```python
from build123d import *

# Parameters (mm, degrees)
SKETCH1_W           = 154
SKETCH1_H           = 100
BOSS_EXTRUDE1_DEPTH = 2
SKETCH2_W           = 100
SKETCH2_H           = 2
BOSS_EXTRUDE2_DEPTH = 70
SKETCH3_W           = 90.6
SKETCH3_H           = 8
BOSS_EXTRUDE3_DEPTH = 8
SKETCH4_W           = 10
SKETCH4_H           = 134
BOSS_EXTRUDE4_DEPTH = 8
SKETCH5_W           = 10
SKETCH5_H           = 5
BOSS_EXTRUDE5_DEPTH = 62
SKETCH6_R           = 1.95
CUT_EXTRUDE1_DEPTH  = 195.889943301
SKETCH7_R           = 1.95
CUT_EXTRUDE2_DEPTH  = 195.889943301
FILLET1_R           = 3
SKETCH8_R           = 1.95
CUT_EXTRUDE3_DEPTH  = 15
SKETCH9_R           = 1.95
CUT_EXTRUDE4_DEPTH  = 15
FILLET2_R           = 3


with BuildPart() as part:
    # Sketch1 → Boss-Extrude1 (new body)
    with BuildSketch(Plane(origin=(0, 0, 0), x_dir=(0, 1, 0), z_dir=(0, 0, 1))):
        with Locations((77, 50)):
            Rectangle(SKETCH1_W, SKETCH1_H)
    extrude(amount=BOSS_EXTRUDE1_DEPTH)

    # Sketch2 → Boss-Extrude2 (add)
    with BuildSketch(Plane.XY.offset(2)):
        with Locations((-50, 153)):
            Rectangle(SKETCH2_W, SKETCH2_H)
        with Locations((-50, 1)):
            Rectangle(SKETCH2_W, SKETCH2_H)
    extrude(amount=BOSS_EXTRUDE2_DEPTH)

    # Sketch3 → Boss-Extrude3 (add)
    with BuildSketch(Plane.XY.offset(2)):
        with Locations((-50, 148)):
            Rectangle(SKETCH3_W, SKETCH3_H)
        with Locations((-50, 6)):
            Rectangle(SKETCH3_W, SKETCH3_H)
    extrude(amount=BOSS_EXTRUDE3_DEPTH)

    # Sketch4 → Boss-Extrude4 (add)
    with BuildSketch(Plane.XY.offset(2)):
        with Locations((-50, 77)):
            Rectangle(SKETCH4_W, SKETCH4_H)
    extrude(amount=BOSS_EXTRUDE4_DEPTH)

    # Sketch5 → Boss-Extrude5 (add)
    with BuildSketch(Plane.XY.offset(10)):
        with Locations((-50, 149.5)):
            Rectangle(SKETCH5_W, SKETCH5_H)
        with Locations((-50, 4.5)):
            Rectangle(SKETCH5_W, SKETCH5_H)
    extrude(amount=BOSS_EXTRUDE5_DEPTH)

    # Sketch6 → Cut-Extrude1 (cut, through all)
    with BuildSketch(Plane(origin=(-95.3, 0, 0), x_dir=(0, -1, 0), z_dir=(-1, 0, 0))):
        with Locations((-6, 6)):
            Circle(SKETCH6_R)
    extrude(amount=-CUT_EXTRUDE1_DEPTH, mode=Mode.SUBTRACT)

    # Sketch7 → Cut-Extrude2 (cut, through all)
    with BuildSketch(Plane(origin=(-95.3, 0, 0), x_dir=(0, -1, 0), z_dir=(-1, 0, 0))):
        with Locations(Location((-148, 6, 0), (0, 0, 90))):
            Circle(SKETCH7_R)
    extrude(amount=-CUT_EXTRUDE2_DEPTH, mode=Mode.SUBTRACT)

    # Fillet1
    fillet1_edges = [part.edges().sort_by_distance(p)[0] for p in [
        (-75.15, 144, 10),
        (-24.85, 10, 10),
        (-75.15, 10, 10),
        (-24.85, 144, 10),
        (-55, 77, 10),
        (-45, 77, 10),
    ]]
    fillet(fillet1_edges, radius=FILLET1_R - 0.0001)  # a hair under: the kernel refuses the full size

    # Sketch8 → Cut-Extrude3 (cut)
    with BuildSketch(Plane.XY.offset(72)):
        with Locations((-50, 150)):
            Circle(SKETCH8_R)
    extrude(amount=-CUT_EXTRUDE3_DEPTH, mode=Mode.SUBTRACT)

    # Sketch9 → Cut-Extrude4 (cut)
    with BuildSketch(Plane.XY.offset(72)):
        with Locations((-50, 4)):
            Circle(SKETCH9_R)
    extrude(amount=-CUT_EXTRUDE4_DEPTH, mode=Mode.SUBTRACT)

    # Fillet2
    fillet2_edges = [part.edges().sort_by_distance(p)[0] for p in [
        (-45, 7, 41),
        (-55, 147, 41),
        (-45, 147, 41),
        (-55, 7, 41),
    ]]
    fillet(fillet2_edges, radius=FILLET2_R)


solid = part.part
```
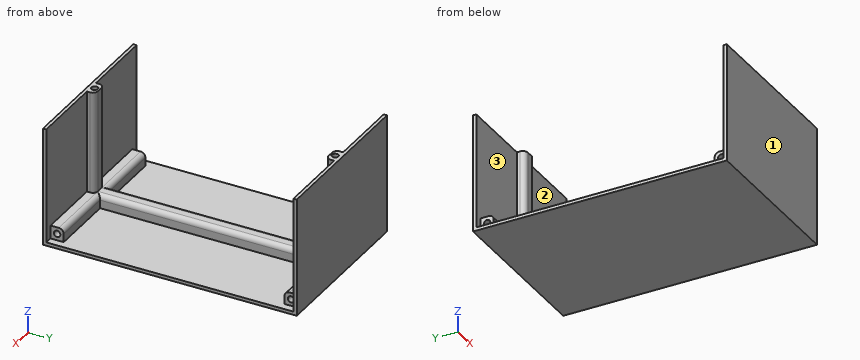
Build history of the part. All positions in model axes, mm. Face numbers are marked on the shaded views. A direction names the side the tool comes from. Round coordinates to 2 decimals unless told otherwise and drop trailing zeros. Order: outer loops, then holes, each group sorted by start corner. A loop starts at its lowest first (then second) coordinate and runs counter-clockwise, first axis right, second up. Notation, with made-up numbers: (-31.75, -37.75) -> (-21.75, -37.75) arc R24 cw to (-21.75, -14.75) -> close; hole circle Ø10 at (81, 36.25). An arc over 180 degrees is marked (long way). Answer in a Markdown table with one row per item.
1) Which spindle directions (+Z, -Z, +X, -X, +Y, -Y) get a long thin tool onto all of the face, cutting with end or side? Do the marked faces 1, 2 and 3. Say none if no direction does.
Values:
| item | result |
|---|---|
| face 1 | +Z, -Z, +X, -X, -Y |
| face 2 | +Z, +X |
| face 3 | +Z, -X |
2) Band-saw the part on B-B on x = -57.5. Give the cut face in (y, z).
Values:
| item | result |
|---|---|
| outline | (0, 0) -> (154, 0) -> (154, 72) -> (152, 72) -> (152, 10) -> (147, 10) arc R3 ccw to (144, 7) -> (144, 2) -> (10, 2) -> (10, 7) arc R3 ccw to (7, 10) -> (2, 10) -> (2, 72) -> (0, 72) -> close; hole circle Ø3.9 at (6, 6); hole circle Ø3.9 at (148, 6) |
3) Band-saw the part on A-A on z = 60.5. Give the cut face in (x, y), and give its area (3 significant figures).
Values:
| item | result |
|---|---|
| outline | (-100, 0) -> (0, 0) -> (0, 2) -> (-45, 2) -> (-45, 4) arc R3 ccw to (-48, 7) -> (-52, 7) arc R3 ccw to (-55, 4) -> (-55, 2) -> (-100, 2) -> close; (-100, 152) -> (-55, 152) -> (-55, 150) arc R3 ccw to (-52, 147) -> (-48, 147) arc R3 ccw to (-45, 150) -> (-45, 152) -> (0, 152) -> (0, 154) -> (-100, 154) -> close; hole circle Ø3.9 at (-50, 4); hole circle Ø3.9 at (-50, 150) |
| area | 468 mm2 |
4) Wall check: L1, parallel to Y at x = -50, z = 63; L2, parallel to Z at x = -37, y = 148; L3, parallel to Y at x = -84.5, z = 35.5. Give the ranges that are in metal, low to high.
Values:
| item | result |
|---|---|
| L1 | 0 to 2.05, 5.95 to 7, 147 to 148.05, 151.95 to 154 |
| L2 | 0 to 4.05, 7.95 to 10 |
| L3 | 0 to 2, 152 to 154 |
5) Pin check, flat tips, straight feed: P1, Ø2, axis at y = 3.5, z = 33.5, coming from the +X side; P2, Ø6, axis at x = -73, y = 54.5, coming from the +Z side; P3, Ø3, axis at y = 148, z = 6, coming from the +X side. Stop position of each tip, or through.
Values:
| item | result |
|---|---|
| P1 | x = -45 |
| P2 | z = 2 |
| P3 | through |
6) Band-saw the part on C-C on z = 18. Give the cut face in (x, y).
Values:
| item | result |
|---|---|
| outline | (-100, 0) -> (0, 0) -> (0, 2) -> (-45, 2) -> (-45, 4) arc R3 ccw to (-48, 7) -> (-52, 7) arc R3 ccw to (-55, 4) -> (-55, 2) -> (-100, 2) -> close; (-100, 152) -> (-55, 152) -> (-55, 150) arc R3 ccw to (-52, 147) -> (-48, 147) arc R3 ccw to (-45, 150) -> (-45, 152) -> (0, 152) -> (0, 154) -> (-100, 154) -> close |
